Here's the drawing with two shaded views (mm, measured from the low corner). I have some questions. A direction names the side the tool comes from. Round coordinates to 2 decimals unless told otherwise and drop trailing zeros. Loops run counter-clockwise (first coordinate to the right, second up) from the corner with the lowest first, then second, coordinate; pieces in that order, holes last. Notation, with made-up numbers: M 20.25,63.5 L 34.25,63.5 A23 cw 34.25,80.5 Z; hole C 82,75 d2. An arc over 180 degrees is marked long. Answer as a JSON object with one key per item and string values.
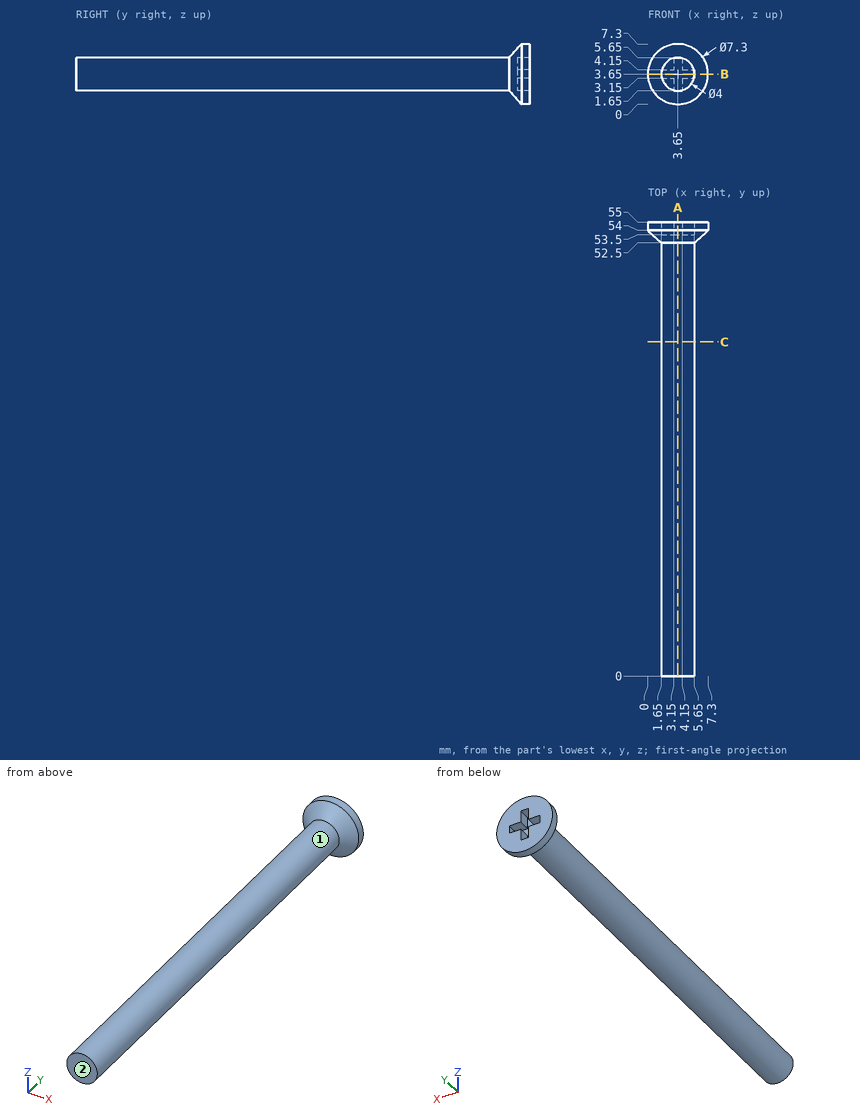
Item 1: For the marked faces 1 and 2, which set-ups out of +Z, -Z, +X, -X, +Y, -Y let a thin tool reach every point of the face, with its end or its side?
Solution:
{"face 1": "-Y", "face 2": "+Z, -Z, +X, -X, -Y"}
Item 2: I want a section at C-C on y = 40.5. List the corners of the cut face in (x, z) for me, plus the area to 3 significant figures.
Solution:
{"outline": "C 3.65,3.65 d4", "area": "12.6 mm2"}
Item 3: If I drill on L1, parallel to Y at x = 4, z = 5; L2, parallel to Z at x = 3.5, y = 9.5; L3, parallel to X at y = 37.5, z = 5, over which ranges is the centre line in solid material (lowest first)? Write a range as from..to.
Solution:
{"L1": "y = 0..53.5", "L2": "z = 1.66..5.64", "L3": "x = 2.17..5.13"}
Item 4: For P1, Ø1.2, axis at x = 2.5, y = 54, coming from the -Z side; P2, Ø2, axis at x = 4, z = 5.5, coming from the +Y side; P3, Ø1.2, axis at x = 2.5, y = 54.5, coming from the +Z side; P4, Ø1.6, axis at x = 5.5, y = 54, coming from the +Z side, each with a flat end and sliding along its axis, tell me the tip position at first contact or that it passes through.
Solution:
{"P1": "stops at z = 0.04", "P2": "stops at y = 55", "P3": "stops at z = 7.26", "P4": "stops at z = 7.15"}
Item 5: I want a section at B-B on z = 3.65. List the corners of the cut face in (x, y) for me.
Solution:
{"outline": "M 0,54 L 1.65,52.5 L 1.65,0 L 5.65,0 L 5.65,52.5 L 7.3,54 L 7.3,55 L 5.65,55 L 5.65,53.5 L 1.65,53.5 L 1.65,55 L 0,55 Z"}
Item 6: I want a section at A-A on x = 3.65. List the corners of the cut face in (y, z) for me.
Solution:
{"outline": "M 0,1.65 L 52.5,1.65 L 54,0 L 55,0 L 55,1.65 L 53.5,1.65 L 53.5,5.65 L 55,5.65 L 55,7.3 L 54,7.3 L 52.5,5.65 L 0,5.65 Z"}
